from build123d import *

# Parameters (mm, degrees)
SKETCH1_R           = 4.5
BOSS_EXTRUDE1_DEPTH = 8


with BuildPart() as part:
    # Sketch1 → Boss-Extrude1 (new body)
    with BuildSketch(Plane.XY):
        with BuildLine():
            Line((-119.390660592, 123.251708428), (-119.390660592, -10.748291572))
            ThreePointArc((-119.390660592, -10.748291572), (-117.047514842, -16.405145821), (-111.390660592, -18.748291572))
            Line((-111.390660592, -18.748291572), (-57.390660592, -18.748291572))
            ThreePointArc((-57.390660592, -18.748291572), (-51.733806343, -21.091437322), (-49.390660592, -26.748291572))
            Line((-49.390660592, -26.748291572), (-49.390660592, -40.748291572))
            ThreePointArc((-49.390660592, -40.748291572), (-47.047514842, -46.405145821), (-41.390660592, -48.748291572))
            Line((-41.390660592, -48.748291572), (149.609339408, -48.748291572))
            ThreePointArc((149.609339408, -48.748291572), (155.266193657, -46.405145821), (157.609339408, -40.748291572))
            Line((157.609339408, -40.748291572), (157.609339408, -23.201759464))
            ThreePointArc((157.609339408, -23.201759464), (156.599247983, -19.310592788), (153.824044881, -16.402034634))
            Line((153.824044881, -16.402034634), (-82.454216652, 130.051433259))
            ThreePointArc((-82.454216652, 130.051433259), (-84.477780716, 130.945790526), (-86.668922126, 131.251708428))
            Line((-86.668922126, 131.251708428), (-111.390660592, 131.251708428))
            ThreePointArc((-111.390660592, 131.251708428), (-117.047514842, 128.908562678), (-119.390660592, 123.251708428))
        make_face()
        with Locations((-99.390660592, 106.251708428)):
            Circle(SKETCH1_R, mode=Mode.SUBTRACT)
        with Locations((-99.390660592, 6.251708428)):
            Circle(SKETCH1_R, mode=Mode.SUBTRACT)
        with Locations((-17.390660592, -33.748291572)):
            Circle(SKETCH1_R, mode=Mode.SUBTRACT)
        with Locations((132.609339408, -33.748291572)):
            Circle(SKETCH1_R, mode=Mode.SUBTRACT)
    extrude(amount=BOSS_EXTRUDE1_DEPTH)


solid = part.part
Geometry: final body of the model. Coordinates: model frame, mm. A direction names the side the tool comes from. Give positions to 0.01 mm unless a question says otherwise; leave off trailing zeros. Write each loop counter-clockwise with the first axis right and the second up, starting at its lowest first coordinate (ties: lowest second). Pieces come first, ordered by that corner, then holes.
(1) Cut plane A-A, the plane z = 5. Return loops of the section in (x, y).
(2) Mould query, pull axis X, two halves, no side actions, for faces 1 (the cylindrical face through (-95.098, 7.603, 3.944)), 2 (the flat face through (-14, 23, 0)), 3 (the flat face through (37.34, 55.8, 3.94)). Classes: released by +X, released by -X, zero draft, split by the parting line, or undercut.
(3) Cut plane B-B, the plane x = 6. Return loops of the section in (y, z).
(4) Cut plane C-C, the plane y = 85. Return loops of the section in (x, z).
(5) Access query for faces 4 (the cylindrical face through (-116.985, 128.97, 3.944)), 5 (the flat face through (-85, -18.748, 4)). Directions: +Z, -Z, +X, -X, +Y, -Y. A direction counts if a zero-diameter tool reaches every point of the face in a straight line with its end or side. Return the directions, or none.
(6) Ray query, line 1 (X direction, y = -33, z = 6); line 2 (X direction, y = -32.5, z = 1.5); line 3 (X direction, y = 114.5, z = 1). Return the intervals inside material, ascending.
(7) First-contact query: P1, Ø5.5, axis at x = -99.39, y = 106.25, coming from the +Z side. Flat tip, straight axial feed; report the tip coordinate or a pass-through.
Values follow:
1. outline: (-119.39, -10.75) arc R8 ccw to (-111.39, -18.75) - (-57.39, -18.75) arc R8 cw to (-49.39, -26.75) - (-49.39, -40.75) arc R8 ccw to (-41.39, -48.75) - (149.61, -48.75) arc R8 ccw to (157.61, -40.75) - (157.61, -23.2) arc R8 ccw to (153.82, -16.4) - (-82.45, 130.05) arc R8 ccw to (-86.67, 131.25) - (-111.39, 131.25) arc R8 ccw to (-119.39, 123.25) - close; hole circle Ø9 at (-99.39, 6.25); hole circle Ø9 at (-99.39, 106.25); hole circle Ø9 at (-17.39, -33.75); hole circle Ø9 at (132.61, -33.75)
2. face 1: undercut
2. face 2: zero draft
2. face 3: released by +X
3. outline: (-48.75, 0) - (75.22, 0) - (75.22, 8) - (-48.75, 8) - close
4. outline: (-119.39, 0) - (-9.77, 0) - (-9.77, 8) - (-119.39, 8) - close
5. face 4: +Z, -Z, -X, +Y
5. face 5: +Z, -Z, -X, -Y
6. line 1: x = -49.39 to -21.83, -12.95 to 128.17, 137.05 to 157.61
6. line 2: x = -49.39 to -21.71, -13.07 to 128.29, 136.93 to 157.61
6. line 3: x = -119.39 to -57.36
7. P1: passes through
